```python
from build123d import *

# Parameters (mm, degrees)
SKETCH1_R           = 12.5
BOSS_EXTRUDE1_DEPTH = 5
SKETCH2_R           = 7.5
BOSS_EXTRUDE2_DEPTH = 20
SKETCH3_R           = 14
BOSS_EXTRUDE3_DEPTH = 9
CHAMFER1_SIZE       = 0.5
CHAMFER1_SIZE2      = 1.5
SKETCH4_R           = 14.5
BOSS_EXTRUDE4_DEPTH = 7
FILLET3_R           = 2
CHAMFER2_SIZE2      = 0.5
CHAMFER2_SIZE       = 0.832139741
CUT_EXTRUDE2_DEPTH  = 6
CIRPATTERN1_COUNT   = 16


with BuildPart() as part:
    # Sketch1 → Boss-Extrude1 (new body)
    with BuildSketch(Plane(origin=(0, 0, 0), x_dir=(1, 0, 0), z_dir=(0, 1, 0))):
        with Locations(Location((0, 0, 0), (0, 0, 270))):
            Circle(SKETCH1_R)
    extrude(amount=BOSS_EXTRUDE1_DEPTH)

    # Sketch2 → Boss-Extrude2 (add)
    with BuildSketch(Plane.XZ):
        with Locations(Location((0, 0, 0), (0, 0, 90))):
            Circle(SKETCH2_R)
    extrude(amount=BOSS_EXTRUDE2_DEPTH)

    # Sketch3 → Boss-Extrude3 (add)
    with BuildSketch(Plane(origin=(0, 5, 0), x_dir=(1, 0, 0), z_dir=(0, 1, 0))):
        with Locations(Location((0, 0, 0), (0, 0, 270))):
            Circle(SKETCH3_R)
    extrude(amount=BOSS_EXTRUDE3_DEPTH)

    # Chamfer1
    chamfer1_edges = [part.edges().sort_by_distance(p)[0] for p in [
        (0, 5, -14),
    ]]
    chamfer1_side = [part.faces().sort_by_distance(p)[0] for p in [
        (0, 5, -13.604020203),
    ]]
    chamfer(chamfer1_edges, length=CHAMFER1_SIZE, length2=CHAMFER1_SIZE2, reference=chamfer1_side[0])

    # Sketch4 → Boss-Extrude4 (add)
    with BuildSketch(Plane(origin=(0, 14, 0), x_dir=(1, 0, 0), z_dir=(0, 1, 0))):
        with Locations(Location((0, 0, 0), (0, 0, 270))):
            Circle(SKETCH4_R)
    extrude(amount=BOSS_EXTRUDE4_DEPTH)

    # Fillet3
    fillet3_edges = [part.edges().sort_by_distance(p)[0] for p in [
        (0, 21, -14.5),
    ]]
    fillet(fillet3_edges, radius=FILLET3_R)

    # Chamfer2
    chamfer2_edges = [part.edges().sort_by_distance(p)[0] for p in [
        (0, 14, -14.5),
    ]]
    chamfer2_side = [part.faces().sort_by_distance(p)[0] for p in [
        (0, 14.01, -14.5),
    ]]
    chamfer(chamfer2_edges, length=CHAMFER2_SIZE - 0.0001, length2=CHAMFER2_SIZE2 - 0.0001, reference=chamfer2_side[0])  # a hair under: the kernel refuses the full size

    # Sketch5 → Cut-Extrude2 (cut)
    with BuildSketch(Plane(origin=(0, 21, 0), x_dir=(1, 0, 0), z_dir=(0, 1, 0))):
        with BuildLine():
            Line((-0.75, 14.5), (0.75, 14.5))
            ThreePointArc((0.75, 14.5), (0, 14.161437828), (-0.75, 14.5))
        make_face()
    cut_extrude2 = extrude(amount=-CUT_EXTRUDE2_DEPTH, mode=Mode.SUBTRACT)

    # CirPattern1: Cut-Extrude2 ×16 about axis
    cirpattern1_axis = Axis((0, 0, 0), (0, 1, 0))
    for i in range(1, CIRPATTERN1_COUNT):
        add(cut_extrude2.rotate(cirpattern1_axis, i * 360 / CIRPATTERN1_COUNT), mode=Mode.SUBTRACT)


solid = part.part
```
Check sheet for the modelled part. Datum: model origin and axes. Units: mm. A direction names the side the tool comes from. Coordinates: 2 decimals unless noted, no trailing zeros. Loops run counter-clockwise (first coordinate to the right, second up) from the corner with the lowest first, then second, coordinate; pieces in that order, holes last.
1) Sectioned sample at D-D (y = 2.5). Record the boundary of the cut face in (x, z).
2) Gauge pin test, flat ends, axial feed: pin 1 (4 mm diameter, centred on x = 7.5, y = 8.5, fed in from -Z); pin 2 (12 mm diameter, centred on y = -13, z = -1.5, fed in from +X); pin 3 (0.5 mm diameter, centred on x = -10, z = 10, fed in from +Y). Record the tip position at first contact, or that the pin passes through.
3) Access from +Z, -Z, +X, -X, +Y, -Y to the whole of each face (thin tool, end or side, straight path). Record for faces 1 (the face through (-5.409, 17.593, -13.088)), 2 (the face through (10.14, 15, -10.13)), 3 (the face through (-10.14, 15, 10.13)), 4 (the face through (-9, 5, 9)), 5 (the face through (5.409, 17.593, 13.088)).
4) Material ranges on probe 1 along Y at (x, z) = (-9.5, 5); probe 2 along Z at (x, y) = (-2, 4); probe 3 along X at (y, z) = (4, 2.5), recorded low to high.
5) Release check for a two-part mould opening along Z. For faces 6 (the face through (3.755, 2.465, 11.923)), 7 (the face through (0.01, 17.59, -14.16)), 8 (the face through (14.16, 17.59, 0.01)) record: released by +Z, released by -Z, zero draft, split by the parting line, or undercut.
Check sheet entries:
1. outline: circle Ø25 at (0, 0)
2. pin 1: stops at z = -12.87
2. pin 2: stops at x = 7.5
2. pin 3: stops at y = 20.44
3. face 1: -Z, +Y
3. face 2: -Z, +X, +Y
3. face 3: +Z, -X, +Y
3. face 4: -Y
3. face 5: +Z, +Y
4. probe 1: y = 0 to 21
4. probe 2: z = -12.34 to 12.34
4. probe 3: x = -12.25 to 12.25
5. face 6: split by the parting line
5. face 7: released by -Z
5. face 8: undercut
